from build123d import *

# Parameters (mm, degrees)
SKETCH004_R     = 4.2
SKETCH004_R_2   = 4.8
SKETCH004_R_3   = 1.518979
SKETCH004_R_4   = 1.54166
SKETCH004_R_5   = 1.514434
SKETCH004_R_6   = 1.53413
SKETCH004_W     = 51.669447
SKETCH004_H     = 40.515184
PAD004_DEPTH    = 6
POCKET_DEPTH    = 4
FILLET002_R     = 1
SKETCH006_R     = 1.977075
SKETCH006_R_2   = 1.924832
SKETCH006_R_3   = 1.937522
SKETCH006_R_4   = 2.033894
POCKET001_DEPTH = 1
SKETCH007_R     = 2.076166
SKETCH007_R_2   = 2.097374
SKETCH007_R_3   = 2.246485
SKETCH007_R_4   = 2.27026
PAD005_DEPTH    = 1


with BuildPart() as part:
    # Sketch004 → Pad004 (new body)
    with BuildSketch(Plane.XY):
        with BuildLine():
            Line((-47.572803, 25.088316), (47.196522, 25.088316))
            add(Edge.make_bspline(
                [(47.196522, 25.088316), (49.583878, 24.67317), (49.843609, 22.181658)],
                knots=[0, 0, 0, 1, 1, 1], degree=2))
            Line((49.843609, 22.181658), (49.843609, -21.958458))
            add(Edge.make_bspline(
                [(49.843609, -21.958458), (49.613785, -24.485321), (46.959763, -24.855799)],
                knots=[0, 0, 0, 1, 1, 1], degree=2))
            Line((46.959763, -24.855799), (-47.489712, -24.855799))
            add(Edge.make_bspline(
                [(-47.489712, -24.855799), (-49.726002, -24.366434), (-50.217018, -22.253706)],
                knots=[0, 0, 0, 1, 1, 1], degree=2))
            Line((-50.217018, -22.253706), (-50.217018, 22.362692))
            add(Edge.make_bspline(
                [(-50.217018, 22.362692), (-49.912418, 24.645672), (-47.572803, 25.088316)],
                knots=[0, 0, 0, 1, 1, 1], degree=2))
        make_face()
        Polygon((-42.563313, 18.368522), (-36.063313, 18.368522), (-36.063313, 11.868522), (-39.313313, 8.618522), (-42.563313, 11.868522), align=None, mode=Mode.SUBTRACT)
        Polygon((-38.898651, 8.147736), (-35.648651, 11.397736), (-29.148651, 11.397736), (-29.148651, 4.897736), (-35.648651, 4.897736), align=None, mode=Mode.SUBTRACT)
        Polygon((-39.254463, 7.585952), (-36.004463, 4.335952), (-36.004463, -2.164048), (-42.504463, -2.164048), (-42.504463, 4.335952), align=None, mode=Mode.SUBTRACT)
        Polygon((-39.610279, 8.14501), (-42.860279, 4.89501), (-49.360279, 4.89501), (-49.360279, 11.39501), (-42.860279, 11.39501), align=None, mode=Mode.SUBTRACT)
        with Locations((-44.968281, -10.264997)):
            Circle(SKETCH004_R, mode=Mode.SUBTRACT)
        with Locations((-33.627011, -10.428595)):
            Circle(SKETCH004_R, mode=Mode.SUBTRACT)
        with Locations((43.730999, 13.356121)):
            Circle(SKETCH004_R_2, mode=Mode.SUBTRACT)
        with Locations((38.86813, 1.894801)):
            Circle(SKETCH004_R_2, mode=Mode.SUBTRACT)
        with Locations((38.891018, -10.470211)):
            Circle(SKETCH004_R, mode=Mode.SUBTRACT)
        with Locations((46.758968, 21.917048)):
            Circle(SKETCH004_R_3, mode=Mode.SUBTRACT)
        with Locations((46.767654, -21.803801)):
            Circle(SKETCH004_R_4, mode=Mode.SUBTRACT)
        with Locations((-47.11446, 21.935822)):
            Circle(SKETCH004_R_5, mode=Mode.SUBTRACT)
        with Locations((-47.138157, -21.794628)):
            Circle(SKETCH004_R_6, mode=Mode.SUBTRACT)
        with Locations((-1.010669, 0.925887)):
            Rectangle(SKETCH004_W, SKETCH004_H, mode=Mode.SUBTRACT)
    extrude(amount=PAD004_DEPTH)

    # Sketch005 (on Face42 of Pad004) → Pocket (cut)
    with BuildSketch(Plane(origin=(0, 0, 0), x_dir=(1, 0, 0), z_dir=(0, 0, -1))):
        Polygon((-49.347778, 15.974498), (-30.138617, 15.974498), (-30.138617, 22.584615), (42.326723, 22.584615), (47.125389, 18.800341), (47.125389, -7.181559), (48.931736, -7.181559), (48.931736, -18.709139), (47.194054, -18.709139), (43.481785, -23.182058), (-43.71611, -23.182058), (-49.347778, -13.90698), align=None)
    extrude(amount=-POCKET_DEPTH, mode=Mode.SUBTRACT)

    # Fillet002
    fillet002_edges = [part.edges().sort_by_distance(p)[0] for p in [
        (-26.845392, 21.183479, 5),
        (-26.845392, -19.331705, 5),
        (24.824055, -19.331705, 5),
        (24.824055, 21.183479, 5),
    ]]
    fillet(fillet002_edges, radius=FILLET002_R)

    # Sketch006 (on Face1 of Fillet002) → Pocket001 (cut)
    with BuildSketch(Plane.XY.offset(6)):
        with Locations((-47.123535, 21.901525)):
            Circle(SKETCH006_R)
        with Locations((46.745956, 21.922697)):
            Circle(SKETCH006_R_2)
        with Locations((46.77578, -21.811125)):
            Circle(SKETCH006_R_3)
        with Locations((-47.121822, -21.801273)):
            Circle(SKETCH006_R_4)
    extrude(amount=-POCKET001_DEPTH, mode=Mode.SUBTRACT)

    # Sketch007 (on Face50 of Pocket001) → Pad005 (join)
    with BuildSketch(Plane.XY.offset(5)):
        with Locations((46.794399, -21.825701)):
            Circle(SKETCH007_R)
        with Locations((46.828327, 21.859865)):
            Circle(SKETCH007_R_2)
        with Locations((-47.145874, 21.87035)):
            Circle(SKETCH007_R_3)
        with Locations((-47.14336, -21.791445)):
            Circle(SKETCH007_R_4)
    extrude(amount=PAD005_DEPTH)


with BuildPart() as part_1:
    # Body001 placement: moved
    add(part.part.moved(Location((0, 0, 1))))


solid = part_1.part
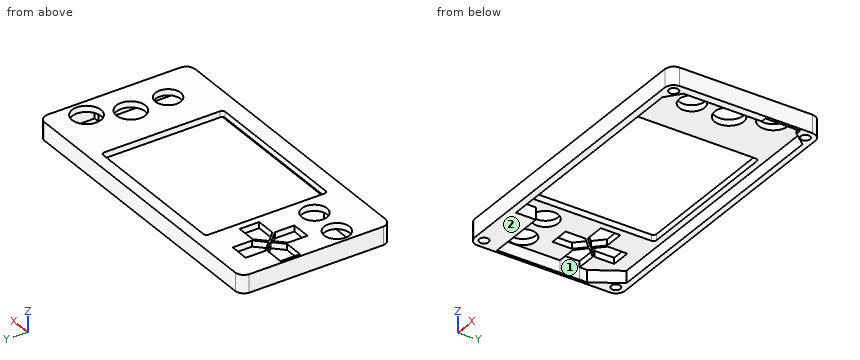
The model under review builds one solid part; all positions refer to its coordinate system, in mm. Face numbers are marked on the shaded views. Round coordinates to 2 decimals unless told otherwise and drop trailing zeros. Loops run counter-clockwise (first coordinate to the right, second up) from the corner with the lowest first, then second, coordinate; pieces in that order, holes last. Notation, with made-up numbers: (-16, 43.25) - (13, 43.25) arc R25 cw to (13, 71.25) - close; hole circle Ø10 at (16, 80.25). An arc over 180 degrees is marked (long way). Use CSV: the item, a comma, the result in double quotes.
(1) For line 1 (X direction, y = 1.5, z = 6.75); line 2 (X direction, y = -18.5, z = 1.5); line 3 (Y direction, x = 21, z = 4), list the stretches that pass through material, from the lowest coordinate up.
Working result:
line 1,"x = -50.22 to -42.5, -36 to -26.85, 24.82 to 34.08, 43.65 to 49.84"
line 2,"x = -50.22 to -30.14, 47.13 to 49.84"
line 3,"y = -24.86 to -22.58, 23.18 to 25.09"
(2) Clearance check with flat-ended pins moving along their axes: P1, Ø11, axis at x = 38.87, y = 1.89, coming from the -Z side; P2, Ø1, axis at x = 24, y = -3.5, coming from the +Z side; P3, Ø1.5, axis at x = 46.5, y = 21.5, coming from the -Z side. State where each tip first meets the part, or that it passes through.
Working result:
P1,"stops at z = 5"
P2,"passes through"
P3,"stops at z = 6"
(3) Take a section at A-A, the plane y = -4. Give the boundary of the cut face in (x, z).
Working result:
outline,"(-50.22, 1) - (-49.35, 1) - (-49.35, 5) - (-26.85, 5) - (-26.85, 7) - (-50.22, 7) - close; (24.82, 5) - (47.13, 5) - (47.13, 1) - (49.84, 1) - (49.84, 7) - (24.82, 7) - close"
(4) Take a section at C-C, the plane y = -13. Give the boundary of the cut face in (x, z), plus the area to 3 significant figures.
Working result:
outline,"(-50.22, 1) - (-49.35, 1) - (-49.35, 5) - (-48.16, 5) - (-48.16, 7) - (-50.22, 7) - close; (-41.78, 5) - (-36.95, 5) - (-36.95, 7) - (-41.78, 7) - close; (-30.31, 5) - (-26.85, 5) - (-26.85, 7) - (-30.31, 7) - close; (24.82, 5) - (35.54, 5) - (35.54, 7) - (24.82, 7) - close; (42.24, 5) - (47.13, 5) - (47.13, 1) - (49.84, 1) - (49.84, 7) - (42.24, 7) - close"
area,"71.7 mm^2"
(5) Take a section at D-D, the plane x = 31.5. Give the boundary of the cut face in (y, z).
Working result:
outline,"(-24.86, 1) - (-22.58, 1) - (-22.58, 5) - (23.18, 5) - (23.18, 1) - (25.09, 1) - (25.09, 7) - (-24.86, 7) - close"
(6) Take a section at B-B, the plane x = 19. Give the boundary of the cut face in (y, z), plus the area to 3 significant figures.
Working result:
outline,"(-24.86, 1) - (-22.58, 1) - (-22.58, 5) - (-19.33, 5) - (-19.33, 7) - (-24.86, 7) - close; (21.18, 5) - (23.18, 5) - (23.18, 1) - (25.09, 1) - (25.09, 7) - (21.18, 7) - close"
area,"35.6 mm^2"
(7) The part is to be moulded in two halves that separate along Y. For the marked faces 1 and 2, say which applies: pulls with the +Y half, pulls with the -Y half, needs draft (parallel to the pull), parting line crosses it, or undercut.
Working result:
face 1,"undercut"
face 2,"needs draft"
